Geometry: final body of the model. Coordinates: model frame, mm. A direction names the side the tool comes from. Coordinates: 2 decimals unless noted, no trailing zeros. Loops run counter-clockwise (first coordinate to the right, second up) from the corner with the lowest first, then second, coordinate; pieces in that order, holes last. Notation, with made-up numbers: (7, 72) - (52, 72) arc R20 ccw to (52, 95) - close; hole circle Ø11 at (-24, 84). An arc over 180 degrees is marked (long way). Answer in a Markdown table with one row per item.
from build123d import *

# Parameters (mm, degrees)
BOSS_EXTRU_1_START = -3
ESQUISSE2_R        = 0.5
BOSS_EXTRU_1_DEPTH = 2


with BuildPart() as part:
    # Esquisse1 → Révolution1 (revolve)
    with BuildSketch(Plane.XY, mode=Mode.PRIVATE) as r_volution1_sk:
        Polygon((-2.4, 0), (-2.4, 3), (-1.15, 3), (-1.15, 4.5), (-2.4, 4.5), (-2.4, 5.5), (-3.7, 5.5), (-3.7, 0), align=None)
    revolve(r_volution1_sk.sketch.rotate(Axis((0, 0, 0), (0, 1, 0)), 270), axis=Axis((0, 0, 0), (0, 1, 0)))

    # Esquisse2 → Boss.-Extru.1 (add)
    with BuildSketch(Plane(origin=(0, 5.5, 0), x_dir=(1, 0, 0), z_dir=(0, 1, 0)).offset(BOSS_EXTRU_1_START)):
        with BuildLine():
            Line((2.165640783, 3), (15.15443587, 1.994028476))
            ThreePointArc((15.15443587, 1.994028476), (17, 0), (15.15443587, -1.994028476))
            Line((15.15443587, -1.994028476), (2.165640783, -3))
            ThreePointArc((2.165640783, -3), (3.7, 0), (2.165640783, 3))
        make_face()
        with Locations(Location((15, 0, 0), (0, 0, 270))):
            Circle(ESQUISSE2_R, mode=Mode.SUBTRACT)
        with Locations(Location((13, 0, 0), (0, 0, 270))):
            Circle(ESQUISSE2_R, mode=Mode.SUBTRACT)
        with Locations(Location((11, 0, 0), (0, 0, 270))):
            Circle(ESQUISSE2_R, mode=Mode.SUBTRACT)
        with Locations(Location((9, 0, 0), (0, 0, 270))):
            Circle(ESQUISSE2_R, mode=Mode.SUBTRACT)
        with Locations(Location((7, 0, 0), (0, 0, 270))):
            Circle(ESQUISSE2_R, mode=Mode.SUBTRACT)
        with Locations(Location((5, 0, 0), (0, 0, 270))):
            Circle(ESQUISSE2_R, mode=Mode.SUBTRACT)
    extrude(amount=BOSS_EXTRU_1_DEPTH)


solid = part.part
(1) Ray query, probe 1 along Y at (x, z) = (4.75, -2); probe 2 along X at (y, z) = (4.75, 1.5); probe 3 along X at (y, z) = (2, 0). Return the intervals inside material, ascending.
Verdict:
| item | result |
|---|---|
| probe 1 | y = 2.5 to 4.5 |
| probe 2 | x = -3.38 to -1.87, 1.87 to 3.38 |
| probe 3 | x = -3.7 to -2.4, 2.4 to 3.7 |
(2) Cut plane B-B on y = 0.7. Output: boundary loops of the cut face in (x, z), then the cut area to 3 significant figures.
Verdict:
| item | result |
|---|---|
| outline | circle Ø7.4 at (0, 0); hole circle Ø4.8 at (0, 0) |
| area | 24.9 mm² |
(3) First-contact query: pin 1 Ø1.5 at (x, y) = (8.5, 3.5) entering from -Z; pin 2 Ø4 at (x, z) = (0, 0) entering from +Y; pin 3 Ø3 at (x, z) = (11.5, -1) entering from -Y. Flat tips, straight axial feed; report the tip coordinate or a pass-through.
Verdict:
| item | result |
|---|---|
| pin 1 | stops at z = -2.57 |
| pin 2 | stops at y = 4.5 |
| pin 3 | stops at y = 2.5 |
(4) Cut plane A-A on x = 0. Output: boundary loops of the cut face in (y, z).
Verdict:
| item | result |
|---|---|
| outline | (0, -3.7) - (5.5, -3.7) - (5.5, -2.4) - (4.5, -2.4) - (4.5, -1.15) - (3, -1.15) - (3, -2.4) - (0, -2.4) - close; (0, 2.4) - (3, 2.4) - (3, 1.15) - (4.5, 1.15) - (4.5, 2.4) - (5.5, 2.4) - (5.5, 3.7) - (0, 3.7) - close |
(5) Access query for faces 4 (the face through (-1, 3, -1)), 5 (the face through (12.556, 3.486, 0.231)), 6 (the face through (-2.024, 5.007, -1.29)). Directions: +Z, -Z, +X, -X, +Y, -Y. A direction counts if a zero-diameter tool reaches every point of the face in a straight line with its end or side. Return the directions, or none.
Verdict:
| item | result |
|---|---|
| face 4 | -Y |
| face 5 | +Y, -Y |
| face 6 | +Y |
(6) Cut plane C-C on z = 0. State how many separate pieces and enclosed holes the cut face has, then the cut area to 4 significant figures.
Verdict:
| item | result |
|---|---|
| separate pieces | 8 |
| enclosed holes | 0 |
| area | 32.65 mm² |
(7) Cut plane D-D on x = 5. Output: boundary loops of the cut face in (y, z).
Verdict:
| item | result |
|---|---|
| outline | (2.5, -2.78) - (4.5, -2.78) - (4.5, -0.5) - (2.5, -0.5) - close; (2.5, 0.5) - (4.5, 0.5) - (4.5, 2.78) - (2.5, 2.78) - close |
(8) Pull-direction query (X, two-part tool) for faces 1 (the face through (5.496, 3.486, -0.065)), 2 (the face through (8.6, 3.5, -2.5)), 3 (the face through (-0.9, 5.5, 2.4)); classes: pulls with the +X half, pulls with the -X half, needs draft (parallel to the pull), parting line crosses it, or undercut.
Verdict:
| item | result |
|---|---|
| face 1 | undercut |
| face 2 | pulls with the +X half |
| face 3 | needs draft |
